```python
from build123d import *

# Parameters (mm, degrees)
SKETCH1_W           = 40
SKETCH1_H           = 40
BOSS_EXTRUDE1_DEPTH = 20
CUT_EXTRUDE1_DEPTH  = 20
CUT_EXTRUDE2_DEPTH  = 10
SKETCH4_W           = 20
SKETCH4_H           = 10
BOSS_EXTRUDE2_DEPTH = 40
CUT_EXTRUDE3_DEPTH  = 40
SKETCH6_W           = 20
SKETCH6_H           = 10
BOSS_EXTRUDE3_DEPTH = 10
BOSS_EXTRUDE4_DEPTH = 10
BOSS_EXTRUDE5_DEPTH = 27
BOSS_EXTRUDE6_DEPTH = 20
CUT_EXTRUDE4_DEPTH  = 20


with BuildPart() as part:
    # Sketch1 → Boss-Extrude1 (new body)
    with BuildSketch(Plane.XY):
        with Locations((20, 20)):
            Rectangle(SKETCH1_W, SKETCH1_H)
    extrude(amount=BOSS_EXTRUDE1_DEPTH)

    # Sketch2 → Cut-Extrude1 (cut)
    with BuildSketch(Plane.XY.offset(20)):
        Polygon((20, 0), (40, 20), (40, 0), align=None)
    extrude(amount=-CUT_EXTRUDE1_DEPTH, mode=Mode.SUBTRACT)

    # Sketch3 → Cut-Extrude2 (cut)
    with BuildSketch(Plane.XY.offset(20)):
        Polygon((30, 20), (30, 10), (40, 20), (40, 30), align=None)
    extrude(amount=-CUT_EXTRUDE2_DEPTH, mode=Mode.SUBTRACT)

    # Sketch4 → Boss-Extrude2 (add)
    with BuildSketch(Plane(origin=(40, 0, 0), x_dir=(0, 0, -1), z_dir=(1, 0, 0))):
        with Locations((-30, 35)):
            Rectangle(SKETCH4_W, SKETCH4_H)
    extrude(amount=-BOSS_EXTRUDE2_DEPTH)

    # Sketch5 → Cut-Extrude3 (cut)
    with BuildSketch(Plane(origin=(0, 30, 0), x_dir=(-1, 0, 0), z_dir=(0, -1, 0))):
        Polygon((-30, -40), (-40, -40), (-40, -30), align=None)
    extrude(amount=-CUT_EXTRUDE3_DEPTH, mode=Mode.SUBTRACT)

    # Sketch6 → Boss-Extrude3 (add)
    with BuildSketch(Plane.ZY):
        with Locations((30, 25)):
            Rectangle(SKETCH6_W, SKETCH6_H)
    extrude(amount=-BOSS_EXTRUDE3_DEPTH)

    # Sketch7 → Boss-Extrude4 (add)
    with BuildSketch(Plane.ZY):
        Polygon((30, 20), (30, 10), (20, 0), (20, 20), align=None)
    extrude(amount=-BOSS_EXTRUDE4_DEPTH)

    # Sketch8 → Boss-Extrude5 (add)
    with BuildSketch(Plane.XY.offset(40)):
        Polygon((10, 20), (20, 30), (10, 30), align=None)
    extrude(amount=-BOSS_EXTRUDE5_DEPTH)

    # Sketch9 → Boss-Extrude6 (add)
    with BuildSketch(Plane.XY.offset(20)):
        Polygon((10, 20), (20, 30), (40, 30), (30, 20), (20, 10), (10, 10), align=None)
    extrude(amount=BOSS_EXTRUDE6_DEPTH)

    # 3DSketch1 → Cut-Extrude4 (cut, along a direction that is not the sketch's normal)
    with BuildSketch(Plane(origin=(20, 30, 40), x_dir=(0.7071067811865471, 0, -0.7071067811865479), z_dir=(-0.5773502691896258, 0.5773502691896264, -0.5773502691896252))):
        Polygon((0, 0), (28.284271247, 0), (14.142135624, 24.494897428), (0, 24.494897428), (-7.071067812, 12.247448714), align=None)
    extrude(amount=-CUT_EXTRUDE4_DEPTH, dir=(-1, 0, 0), mode=Mode.SUBTRACT)


with BuildPart() as body_2:
    # of the pieces the cut leaves, the one that is kept (cut_extrude4_keep)
    add(part.part.solids().sort_by_distance((0, 0, 0))[0])


solid = body_2.part
```
For this review, take the finished solid that the model builds, in its own axes (mm). A direction names the side the tool comes from. Round coordinates to 2 decimals unless told otherwise and drop trailing zeros. Write each loop counter-clockwise with the first axis right and the second up, starting at its lowest first coordinate (ties: lowest second). Pieces come first, ordered by that corner, then holes. Notation, with made-up numbers: (6.5, 69) -> (55.5, 69) arc R16 ccw to (55.5, 97) -> close; hole circle Ø5 at (34.5, 81). An arc over 180 degrees is marked (long way). One line per question, with ' | ' between items. Start each with the question number.
1) For pin 1 Ø5 at (x, y) = (36.5, 16) entering from +Z; pin 2 Ø11 at (y, z) = (16, 16) entering from +X; pin 3 Ø5 at (x, z) = (15.5, 24.5) entering from -Y, all flat-tipped, find the tip position at first contact; note any pin that passes through.
2) Machinability: for faces 1 (the flat face through (5, 20, 35)), 2 (the flat face through (5, 5, 25)), 3 (the flat face through (35, 25, 15)), which of the approach directions +Z, -Z, +X, -X, +Y, -Y give a long, thin tool a straight path to every point of the face, cutting with its end or side? Answer none if there is none.
3) Add section A-A (x = 22.5). Write out the cut boundary in (y, z), and give its area (3 significant figures).
4) Add section B-B (y = 13.5). Write out the cut boundary in (x, z).
5) Add section D-D (x = 31). Write out the cut boundary in (y, z).
6) Add section C-C (z = 24). Write out the cut boundary in (x, y), and give its area (3 significant figures).
7) Wall thickness on line 1 along X through (y, z) = (9.5, 26); line 2 along Z through (x, y) = (6, 18): over which ranges is each line inside the solid? List them lowest first.
Reported:
1) pin 1: stops at z = 10 | pin 2: stops at x = 31.5 | pin 3: stops at y = 10
2) face 1: +Z, -X, -Y | face 2: +Z, +X, -X, -Y | face 3: +Z, +X, -Y
3) outline: (2.5, 0) -> (40, 0) -> (40, 40) -> (30, 40) -> (30, 37.5) -> (12.5, 20) -> (2.5, 20) -> close | area: 1,100 mm²
4) outline: (0, 0) -> (33.5, 0) -> (33.5, 10) -> (30, 10) -> (30, 20) -> (23.5, 20) -> (10, 33.5) -> (10, 30) -> (0, 30) -> close
5) outline: (11, 0) -> (40, 0) -> (40, 39) -> (30, 39) -> (30, 29) -> (21, 20) -> (21, 10) -> (11, 10) -> close
6) outline: (0, 4) -> (10, 4) -> (10, 10) -> (16, 10) -> (36, 30) -> (40, 30) -> (40, 40) -> (0, 40) -> close | area: 980 mm²
7) line 1: x = 0 to 10 | line 2: z = 0 to 30
